from build123d import *

# Parameters (mm, degrees)
BOSS_EXTRU_1_DEPTH      = 8
ESQUISSE2_R             = 2.45
ENL_V_MAT_EXTRU_1_DEPTH = 3
ENL_V_MAT_EXTRU_2_REACH = 7
ESQUISSE3_R             = 1.25
ESQUISSE4_R             = 3
ENL_V_MAT_EXTRU_3_DEPTH = 2
ENL_V_MAT_EXTRU_4_DEPTH = 4


with BuildPart() as part:
    # Esquisse1 → Boss.-Extru.1 (new body)
    with BuildSketch(Plane(origin=(0, 0, 0), x_dir=(1, 0, 0), z_dir=(0, 1, 0))):
        with BuildLine():
            Line((-3, 26.381049961), (-3, 4.963869458))
            ThreePointArc((-3, 4.963869458), (0, -5.8), (3, 4.963869458))
            Line((3, 4.963869458), (3, 38.463869458))
            Line((3, 38.463869458), (-0.867157449, 56.657414832))
            Line((-0.867157449, 56.657414832), (-1.84530505, 56.449503141))
            ThreePointArc((-1.84530505, 56.449503141), (-3.756758837, 55.119060789), (-4.140414176, 52.821988519))
            Line((-4.140414176, 52.821988519), (-3, 49.618950039))
            ThreePointArc((-3, 49.618950039), (0, 38), (-3, 26.381049961))
        make_face()
    extrude(amount=BOSS_EXTRU_1_DEPTH)

    # Esquisse2 → Enlèv. mat.-Extru.1 (cut)
    with BuildSketch(Plane(origin=(0, 8, 0), x_dir=(1, 0, 0), z_dir=(0, 1, 0))):
        Circle(ESQUISSE2_R)
    extrude(amount=-ENL_V_MAT_EXTRU_1_DEPTH, mode=Mode.SUBTRACT)

    # Esquisse3 → Enlèv. mat.-Extru.2 (cut, up to next)
    with BuildSketch(Plane(origin=(0, 5, 0), x_dir=(1, 0, 0), z_dir=(0, 1, 0)), mode=Mode.PRIVATE) as enl_v_mat_extru_2_sk1:
        Circle(ESQUISSE3_R)
    enl_v_mat_extru_2_tool1 = extrude(enl_v_mat_extru_2_sk1.sketch, amount=-ENL_V_MAT_EXTRU_2_REACH, mode=Mode.PRIVATE) & part.part
    add(enl_v_mat_extru_2_tool1.solids().sort_by_distance((0, 5, 0))[0], mode=Mode.SUBTRACT)

    # Esquisse4 → Enlèv. mat.-Extru.3 (cut)
    with BuildSketch(Plane.XZ):
        Circle(ESQUISSE4_R)
    extrude(amount=-ENL_V_MAT_EXTRU_3_DEPTH, mode=Mode.SUBTRACT)

    # Esquisse5 → Enlèv. mat.-Extru.4 (cut)
    with BuildSketch(Plane(origin=(0, 8, 0), x_dir=(1, 0, 0), z_dir=(0, 1, 0))):
        with BuildLine():
            Line((-3, 4.963869458), (-3, 17.24093965))
            ThreePointArc((-3, 17.24093965), (0, 17.5), (3, 17.24093965))
            Line((3, 17.24093965), (3, 4.963869458))
            ThreePointArc((3, 4.963869458), (0, 5.8), (-3, 4.963869458))
        make_face()
    extrude(amount=-ENL_V_MAT_EXTRU_4_DEPTH, mode=Mode.SUBTRACT)


solid = part.part
The model under review builds one solid part; all positions refer to its coordinate system, in mm. A direction names the side the tool comes from. Give positions to 0.01 mm unless a question says otherwise; leave off trailing zeros. Order: outer loops, then holes, each group sorted by start corner. A loop starts at its lowest first (then second) coordinate and runs counter-clockwise, first axis right, second up. Notation, with made-up numbers: (62.25, 28) -> (110.25, 28) arc R14 ccw to (110.25, 44) -> close; hole circle Ø7 at (64.5, -6). An arc over 180 degrees is marked (long way). Write item = value, one per line. Start each with the question number.
(1) Tool access review of faces 4 (the flat face through (-3, 3, -18)), 5 (the cylindrical face through (0, 6, -17.5)), 6 (the flat face through (3, 4, -25)), 7 (the flat face through (1, 2, -1)): name each direction out of +Z, -Z, +X, -X, +Y, -Y from which nothing blocks a thin tool from reaching the whole face with its end or side.
(2) Take a section at C-C (z = 0). Write out the cut boundary in (x, y), plus the area to 3 significant figures.
(3) For L1, parallel to X at y = 7.35, z = 0; L2, parallel to Z at x = -2, y = 1; L3, parallel to X at y = 3.3, z = 0, list the stretches that pass through material, from the lowest coordinate up. Write a range as from..to.
(4) Take a section at B-B (y = 1). Write out the cut boundary in (x, z), plus the area to 3 significant figures.
(5) Take a section at D-D (x = 4.5). Write out the cut boundary in (y, z), plus the area to 3 significant figures.
(6) For pin 1 Ø1.5 at (y, z) = (6, -36) entering from -X; pin 2 Ø1.8 at (x, z) = (-0.5, -10.5) entering from +Y; pin 3 Ø4 at (y, z) = (6.5, -41.5) entering from +X, all flat-tipped, find the tip position at first contact; note any pin that passes through.
(7) Draft analysis for pull direction Z (two halves, no side actions). For faces 1 (the flat face through (-3.578, 3.944, -51.243)), 2 (the flat face through (0.14, 8, -37.23)), 3 (the flat face through (1.1, 3.9, -47.4)), state which applies: +Z half, -Z half, draft (parallel to the pull), parting line (faces both ways), or undercut.
(8) Take a section at A-A (y = 7). Write out the cut boundary in (x, z), plus the area to 3 significant figures.
Returned:
q1.face_4 = -X, +Y, -Y
q1.face_5 = +Y
q1.face_6 = -Z, +X, +Y, -Y
q1.face_7 = -Y
q2.outline = (-5.8, 0) -> (-3, 0) -> (-3, 2) -> (-1.25, 2) -> (-1.25, 5) -> (-2.45, 5) -> (-2.45, 8) -> (-5.8, 8) -> close; (1.25, 2) -> (3, 2) -> (3, 0) -> (5.8, 0) -> (5.8, 8) -> (2.45, 8) -> (2.45, 5) -> (1.25, 5) -> close
q2.area = 58.6 mm²
q3.L1 = -5.8..-2.45, 2.45..5.8
q3.L2 = -56.41..-47.59, -28.41..-2.24, 2.24..5.44
q3.L3 = -5.8..-1.25, 1.25..5.8
q4.outline = (-4.14, -52.82) arc R3 ccw to (-1.85, -56.45) -> (-0.87, -56.66) -> (3, -38.46) -> (3, -4.96) arc R5.8 ccw (long way) to (-3, -4.96) -> (-3, -26.38) arc R24 cw to (-3, -49.62) -> close; hole circle Ø6 at (0, 0)
q4.area = 306 mm²
q5.outline = (0, -3.66) -> (8, -3.66) -> (8, 3.66) -> (0, 3.66) -> close
q5.area = 58.5 mm²
q6.pin_1 = -0.16
q6.pin_2 = 4
q6.pin_3 = 2.78
q7.face_1 = undercut
q7.face_2 = draft
q7.face_3 = -Z half
q8.outline = circle Ø11.6 at (0, 0); (-4.14, -52.82) arc R3 ccw to (-1.85, -56.45) -> (-0.87, -56.66) -> (3, -38.46) -> (3, -17.24) arc R17.5 cw to (-3, -17.24) -> (-3, -26.38) arc R24 cw to (-3, -49.62) -> close; hole circle Ø4.9 at (0, 0)
q8.area = 244 mm²
